Can you work these out from the model? Positions are in its coordinate system, mm. A direction names the side the tool comes from. Give positions to 0.01 mm unless a question says otherwise; leave off trailing zeros. Loops run counter-clockwise (first coordinate to the right, second up) from the corner with the lowest first, then second, coordinate; pieces in that order, holes last. Notation, with made-up numbers: (60.25, 41.5) - (72.25, 41.5) arc R20 cw to (72.25, 64.5) - close; hole circle Ø4 at (24, 53). An arc over 180 degrees is marked (long way). Answer as a JSON object with one key per item and string values.
```python
from build123d import *

# Parameters (mm, degrees)
CROQUIS1_W              = 150
CROQUIS1_H              = 135
SALIENTE_EXTRUIR1_DEPTH = 2
CORTAR_EXTRUIR2_DEPTH   = 2
CROQUIS4_W              = 150
CROQUIS4_H              = 135
CROQUIS4_W_2            = 146
CROQUIS4_H_2            = 131
SALIENTE_EXTRUIR3_DEPTH = 72
CROQUIS5_R              = 1.5
CORTAR_EXTRUIR3_DEPTH   = 2
CROQUIS6_R              = 1.5
CORTAR_EXTRUIR4_DEPTH   = 2
CROQUIS7_R              = 1.5
CORTAR_EXTRUIR5_DEPTH   = 2
CROQUIS8_R              = 1.43177866
CORTAR_EXTRUIR6_DEPTH   = 2
CROQUIS9_W              = 10
CROQUIS9_H              = 10
CORTAR_EXTRUIR7_DEPTH   = 2
CROQUIS10_W             = 10
CROQUIS10_H             = 10
CORTAR_EXTRUIR8_DEPTH   = 2
CROQUIS11_W             = 10
CROQUIS11_H             = 10
CROQUIS11_W_2           = 19
CROQUIS11_H_2           = 40
CORTAR_EXTRUIR9_DEPTH   = 2
CROQUIS13_R             = 2
CORTAR_EXTRUIR11_DEPTH  = 2
CROQUIS14_W             = 10
CROQUIS14_H             = 10
CROQUIS14_R             = 2
SALIENTE_EXTRUIR4_DEPTH = 5
CROQUIS15_W             = 5
CROQUIS15_H             = 4
CROQUIS15_W_2           = 40
CROQUIS15_H_2           = 3
CORTAR_EXTRUIR12_DEPTH  = 2
CROQUIS12_W             = 15
CROQUIS12_H             = 15
CORTAR_EXTRUIR13_DEPTH  = 2
SALIENTE_EXTRUIR5_DEPTH = 74
SALIENTE_EXTRUIR6_DEPTH = 27.2
SALIENTE_EXTRUIR7_REACH = 123.232


with BuildPart() as part:
    # Croquis1 → Saliente-Extruir1 (new body)
    with BuildSketch(Plane(origin=(0, 0, 0), x_dir=(1, 0, 0), z_dir=(0, 1, 0))):
        Rectangle(CROQUIS1_W, CROQUIS1_H)
    extrude(amount=SALIENTE_EXTRUIR1_DEPTH)

    # Croquis2 → Cortar-Extruir2 (cut)
    with BuildSketch(Plane(origin=(0, 2, 0), x_dir=(1, 0, 0), z_dir=(0, 1, 0))):
        with BuildLine():
            Line((31.25, 16.5), (31.25, 1.5))
            Line((31.25, 1.5), (16.25, 1.5))
            ThreePointArc((16.25, 1.5), (14.75, 0), (16.25, -1.5))
            Line((16.25, -1.5), (31.25, -1.5))
            Line((31.25, -1.5), (31.25, -16.5))
            ThreePointArc((31.25, -16.5), (32.75, -18), (34.25, -16.5))
            Line((34.25, -16.5), (34.25, -1.5))
            Line((34.25, -1.5), (49.25, -1.5))
            ThreePointArc((49.25, -1.5), (50.75, 0), (49.25, 1.5))
            Line((49.25, 1.5), (34.25, 1.5))
            Line((34.25, 1.5), (34.25, 16.5))
            ThreePointArc((34.25, 16.5), (32.75, 18), (31.25, 16.5))
        make_face()
        with BuildLine():
            Line((-31.25, -16.5), (-31.25, -1.5))
            Line((-31.25, -1.5), (-16.25, -1.5))
            ThreePointArc((-16.25, -1.5), (-14.75, 0), (-16.25, 1.5))
            Line((-16.25, 1.5), (-31.25, 1.5))
            Line((-31.25, 1.5), (-31.25, 16.5))
            ThreePointArc((-31.25, 16.5), (-32.75, 18), (-34.25, 16.5))
            Line((-34.25, 16.5), (-34.25, 1.5))
            Line((-34.25, 1.5), (-49.25, 1.5))
            ThreePointArc((-49.25, 1.5), (-50.75, 0), (-49.25, -1.5))
            Line((-49.25, -1.5), (-34.25, -1.5))
            Line((-34.25, -1.5), (-34.25, -16.5))
            ThreePointArc((-34.25, -16.5), (-32.75, -18), (-31.25, -16.5))
        make_face()
    extrude(amount=-CORTAR_EXTRUIR2_DEPTH, mode=Mode.SUBTRACT)

    # Croquis4 → Saliente-Extruir3 (add)
    with BuildSketch(Plane(origin=(0, 2, 0), x_dir=(1, 0, 0), z_dir=(0, 1, 0))):
        Rectangle(CROQUIS4_W, CROQUIS4_H)
        Rectangle(CROQUIS4_W_2, CROQUIS4_H_2, mode=Mode.SUBTRACT)
    extrude(amount=SALIENTE_EXTRUIR3_DEPTH)

    # Croquis5 → Cortar-Extruir3 (cut)
    with BuildSketch(Plane.ZY.offset(75)):
        with Locations((-60.5, 69)):
            Circle(CROQUIS5_R)
    extrude(amount=-CORTAR_EXTRUIR3_DEPTH, mode=Mode.SUBTRACT)

    # Croquis6 → Cortar-Extruir4 (cut)
    with BuildSketch(Plane.ZY.offset(75)):
        with Locations((60.5, 69)):
            Circle(CROQUIS6_R)
    extrude(amount=-CORTAR_EXTRUIR4_DEPTH, mode=Mode.SUBTRACT)

    # Croquis7 → Cortar-Extruir5 (cut)
    with BuildSketch(Plane(origin=(75, 0, 0), x_dir=(0, 0, -1), z_dir=(1, 0, 0))):
        with Locations((56.5, 69)):
            Circle(CROQUIS7_R)
    extrude(amount=-CORTAR_EXTRUIR5_DEPTH, mode=Mode.SUBTRACT)

    # Croquis8 → Cortar-Extruir6 (cut)
    with BuildSketch(Plane(origin=(75, 0, 0), x_dir=(0, 0, -1), z_dir=(1, 0, 0))):
        with Locations((-60.5, 69)):
            Circle(CROQUIS8_R)
    extrude(amount=-CORTAR_EXTRUIR6_DEPTH, mode=Mode.SUBTRACT)

    # Croquis9 → Cortar-Extruir7 (cut)
    with BuildSketch(Plane.XY.offset(67.5)):
        with Locations((-2, 53.8)):
            Rectangle(CROQUIS9_W, CROQUIS9_H)
        with Locations((-55, 53.8)):
            Rectangle(CROQUIS9_W, CROQUIS9_H)
        with Locations((-37, 53.8)):
            Rectangle(CROQUIS9_W, CROQUIS9_H)
        with Locations((-20, 53.8)):
            Rectangle(CROQUIS9_W, CROQUIS9_H)
        with Locations((16, 53.8)):
            Rectangle(CROQUIS9_W, CROQUIS9_H)
        with Locations((34, 53.8)):
            Rectangle(CROQUIS9_W, CROQUIS9_H)
        with Locations((53, 53.8)):
            Rectangle(CROQUIS9_W, CROQUIS9_H)
    extrude(amount=-CORTAR_EXTRUIR7_DEPTH, mode=Mode.SUBTRACT)

    # Croquis10 → Cortar-Extruir8 (cut)
    with BuildSketch(Plane(origin=(75, 0, 0), x_dir=(0, 0, -1), z_dir=(1, 0, 0))):
        with Locations((16.5, 53.8)):
            Rectangle(CROQUIS10_W, CROQUIS10_H)
        with Locations((-39.5, 53.8)):
            Rectangle(CROQUIS10_W, CROQUIS10_H)
        with Locations((-19.5, 53.8)):
            Rectangle(CROQUIS10_W, CROQUIS10_H)
        with Locations((0.5, 53.8)):
            Rectangle(CROQUIS10_W, CROQUIS10_H)
        with Locations((32.5, 53.8)):
            Rectangle(CROQUIS10_W, CROQUIS10_H)
        with Locations((47.5, 53.8)):
            Rectangle(CROQUIS10_W, CROQUIS10_H)
    extrude(amount=-CORTAR_EXTRUIR8_DEPTH, mode=Mode.SUBTRACT)

    # Croquis11 → Cortar-Extruir9 (cut)
    with BuildSketch(Plane(origin=(0, 0, -67.5), x_dir=(-1, 0, 0), z_dir=(0, 0, -1))):
        with Locations((-5, 53.8)):
            Rectangle(CROQUIS11_W, CROQUIS11_H)
        with Locations((15.5, 26.8)):
            Rectangle(CROQUIS11_W_2, CROQUIS11_H_2)
        with Locations((40.5, 26.8)):
            Rectangle(CROQUIS11_W_2, CROQUIS11_H_2)
        with Locations((63.5, 26.8)):
            Rectangle(CROQUIS11_W_2, CROQUIS11_H_2)
    extrude(amount=-CORTAR_EXTRUIR9_DEPTH, mode=Mode.SUBTRACT)

    # Croquis13 → Cortar-Extruir11 (cut)
    with BuildSketch(Plane.XZ):
        with Locations(Location((-26, 38, 0), (0, 0, 270))):
            Circle(CROQUIS13_R)
        with Locations(Location((26, 38, 0), (0, 0, 90))):
            Circle(CROQUIS13_R)
    extrude(amount=-CORTAR_EXTRUIR11_DEPTH, mode=Mode.SUBTRACT)

    # Croquis14 → Saliente-Extruir4 (add)
    # profile 1 of 2: a face of its own
    with BuildSketch(Plane(origin=(0, 2, 0), x_dir=(1, 0, 0), z_dir=(0, 1, 0))):
        with Locations((26, -38)):
            Rectangle(CROQUIS14_W, CROQUIS14_H)
        with Locations(Location((26, -38, 0), (0, 0, 270))):
            Circle(CROQUIS14_R, mode=Mode.SUBTRACT)
    # profile 2 of 2: a face of its own
    with BuildSketch(Plane(origin=(0, 2, 0), x_dir=(1, 0, 0), z_dir=(0, 1, 0))):
        with Locations((-26, -38)):
            Rectangle(CROQUIS14_W, CROQUIS14_H)
        with Locations(Location((-26, -38, 0), (0, 0, 90))):
            Circle(CROQUIS14_R, mode=Mode.SUBTRACT)
    extrude(amount=SALIENTE_EXTRUIR4_DEPTH)

    # Croquis15 → Cortar-Extruir12 (cut)
    with BuildSketch(Plane.XY.offset(67.5)):
        with Locations((0, 4)):
            Rectangle(CROQUIS15_W, CROQUIS15_H)
        with Locations((0, 13.5)):
            Rectangle(CROQUIS15_W_2, CROQUIS15_H_2)
        with Locations((0, 20.5)):
            Rectangle(CROQUIS15_W_2, CROQUIS15_H_2)
        with Locations((0, 27.5)):
            Rectangle(CROQUIS15_W_2, CROQUIS15_H_2)
    extrude(amount=-CORTAR_EXTRUIR12_DEPTH, mode=Mode.SUBTRACT)

    # Croquis12 → Cortar-Extruir13 (cut)
    with BuildSketch(Plane(origin=(75, 0, 0), x_dir=(0, 0, -1), z_dir=(1, 0, 0))):
        with Locations((18, 66.3)):
            Rectangle(CROQUIS12_W, CROQUIS12_H)
        with Locations((-13, 66.3)):
            Rectangle(CROQUIS12_W, CROQUIS12_H)
    extrude(amount=-CORTAR_EXTRUIR13_DEPTH, mode=Mode.SUBTRACT)

    # Croquis16 → Saliente-Extruir5 (add)
    with BuildSketch(Plane(origin=(0, 74, 0), x_dir=(1, 0, 0), z_dir=(0, 1, 0))):
        Polygon((-73, -65.5), (-73, -63.5), (-71, -65.5), align=None)
        Polygon((73, -65.5), (71, -65.5), (73, -63.5), align=None)
        Polygon((73, 65.5), (73, 63.5), (71, 65.5), align=None)
    extrude(amount=-SALIENTE_EXTRUIR5_DEPTH)

    # Croquis17 → Saliente-Extruir6 (add)
    with BuildSketch(Plane(origin=(0, 74, 0), x_dir=(1, 0, 0), z_dir=(0, 1, 0))):
        Polygon((-73, 65.5), (-73, 63.5), (-71, 65.5), align=None)
    extrude(amount=-SALIENTE_EXTRUIR6_DEPTH)

    # Croquis18 → Saliente-Extruir7 (add, up to next)
    with BuildSketch(Plane(origin=(0, 6.8, 0), x_dir=(1, 0, 0), z_dir=(0, 1, 0)), mode=Mode.PRIVATE) as saliente_extruir7_sk1:
        Polygon((-73, 65.5), (-71, 65.5), (-73, 63.5), align=None)
    saliente_extruir7_tool1 = extrude(saliente_extruir7_sk1.sketch, amount=-SALIENTE_EXTRUIR7_REACH, mode=Mode.PRIVATE) - part.part
    add(saliente_extruir7_tool1.solids().sort_by_distance((-72.333333, 6.8, -64.833333))[0])


solid = part.part
```
1) Imagine slicing it at A-A on y = 38.5. Write out the boundary of the cut face in (x, z), and give its area (3 significant figures).
Check sheet entries:
{"outline": "(-75, -67.5) - (-73, -67.5) - (-73, 63.5) - (-71, 65.5) - (71, 65.5) - (73, 63.5) - (73, -63.5) - (71, -65.5) - (-6, -65.5) - (-6, -67.5) - (75, -67.5) - (75, 67.5) - (-75, 67.5) - close; (-54, -67.5) - (-50, -67.5) - (-50, -65.5) - (-54, -65.5) - close; (-31, -67.5) - (-25, -67.5) - (-25, -65.5) - (-31, -65.5) - close", "area": "1,020 mm2"}
2) Which directions (+Z, -Z, +X, -X, +Y, -Y) give clear straight access to the entire face, cutting with the end or side of a thin tool? Please do faces 1 (the flat face through (-64, 46.8, -66)), 2 (the flat face through (-26, 4, 43)), 3 (the flat face through (1, 0, -1)).
Check sheet entries:
{"face 1": "-Z", "face 2": "+Y", "face 3": "+Z, -Z, +X, -X, -Y"}
3) I need wall thicknesses on L1, parallel to Z at x = -26, y = 3.25; L2, parallel to X at y = 3.35, z = 38; L3, parallel to Z at x = 73.7, y = 69. Which ranges of each line are inside material? Lowest first, please.
Check sheet entries:
{"L1": "-67.5 to -65.5, 33 to 36, 40 to 43, 65.5 to 67.5", "L2": "-75 to -73, -31 to -28, -24 to -21, 21 to 24, 28 to 31, 73 to 75", "L3": "-67.5 to -58, -55 to -25.5, -10.5 to 5.5, 20.5 to 59.07, 61.93 to 67.5"}
4) If we mould it in two halves opening along Z, with no side actions, what happens to faces 4 (the flat face through (-1, 36, 67.5)), 5 (the flat face through (-21, 4, 38)), 6 (the flat face through (-75, 36, 1))? For each: released by +Z, released by -Z, zero draft, split by the parting line, or undercut.
Check sheet entries:
{"face 4": "released by +Z", "face 5": "undercut", "face 6": "zero draft"}
5) Imagine slicing it at D-D on x = 26. Write out the boundary of the cut face in (y, z), and give its area (3 significant figures).
Check sheet entries:
{"outline": "(0, -67.5) - (74, -67.5) - (74, -65.5) - (2, -65.5) - (2, -1.5) - (0, -1.5) - close; (0, 1.5) - (2, 1.5) - (2, 33) - (7, 33) - (7, 36) - (0, 36) - close; (0, 40) - (7, 40) - (7, 43) - (2, 43) - (2, 65.5) - (74, 65.5) - (74, 67.5) - (0, 67.5) - close", "area": "574 mm2"}
6) Imagine slicing it at B-B on z = 38. Write out the boundary of the cut face in (x, y).
Check sheet entries:
{"outline": "(-75, 0) - (-28, 0) - (-28, 7) - (-31, 7) - (-31, 2) - (-73, 2) - (-73, 74) - (-75, 74) - close; (-24, 0) - (24, 0) - (24, 7) - (21, 7) - (21, 2) - (-21, 2) - (-21, 7) - (-24, 7) - close; (28, 0) - (75, 0) - (75, 48.8) - (73, 48.8) - (73, 2) - (31, 2) - (31, 7) - (28, 7) - close; (73, 58.8) - (75, 58.8) - (75, 74) - (73, 74) - close"}
7) Imagine slicing it at C-C on x = -13. Write out the boundary of the cut face in (y, z).
Check sheet entries:
{"outline": "(0, -67.5) - (6.8, -67.5) - (6.8, -65.5) - (2, -65.5) - (2, 65.5) - (12, 65.5) - (12, 67.5) - (0, 67.5) - close; (15, 65.5) - (19, 65.5) - (19, 67.5) - (15, 67.5) - close; (22, 65.5) - (26, 65.5) - (26, 67.5) - (22, 67.5) - close; (29, 65.5) - (74, 65.5) - (74, 67.5) - (29, 67.5) - close; (46.8, -67.5) - (74, -67.5) - (74, -65.5) - (46.8, -65.5) - close"}
